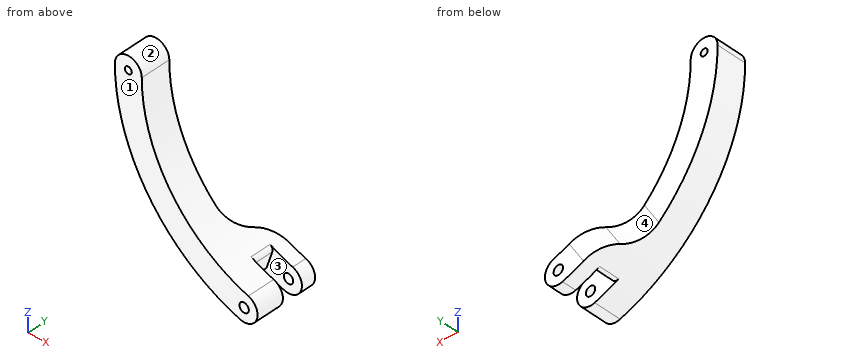
from build123d import *

# Parameters (mm, degrees)
SKETCH1_R               = 0.7499999999999986
SKETCH1_R_2             = 1.0249999999999995
BOSS_EXTRUDE1_DEPTH     = 6.510019999999999
BOSS_EXTRU_1_DEPTH      = 7.112
CONG_1_R                = 7.112
CONG_2_R                = 6.35
ENL_V_MAT_EXTRU_1_DEPTH = 4.444999999999999
ESQUISSE4_R             = 1.024999999999998
ENL_V_MAT_EXTRU_2_DEPTH = 57.18027536353634
CONG_3_R                = 1.016


with BuildPart() as part:
    # Sketch1 → Boss-Extrude1 (new body)
    with BuildSketch(Plane(origin=(0, 0, 0), x_dir=(1, 0, 0), z_dir=(0, 1, 0))):
        with BuildLine():
            ThreePointArc((-33.59051080682659, 0), (-27.195497439499345, 19.716169386615615), (-10.445442396451748, 31.92514916810793))
            ThreePointArc((-10.445442396451748, 31.92514916810793), (-8.576954256445317, 35.61090468912391), (-12.262709777461287, 37.4793928291303))
            ThreePointArc((-12.262709777461287, 37.4793928291303), (-31.926890187777666, 23.14633061338439), (-39.43448919317339, 0))
            ThreePointArc((-39.43448919317339, 0), (-36.512499999999996, -2.9219891931734026), (-33.59051080682659, 0))
        make_face()
        with Locations(Location((-36.512499999999996, 0, 0), (0, 0, 270))):
            Circle(SKETCH1_R, mode=Mode.SUBTRACT)
        with Locations(Location((-11.354076086956523, 34.702270998619134, 0), (0, 0, 270))):
            Circle(SKETCH1_R_2, mode=Mode.SUBTRACT)
    extrude(amount=BOSS_EXTRUDE1_DEPTH)

    # Esquisse1 → Boss.-Extru.1 (add)
    with BuildSketch(Plane(origin=(0, 6.510019999999999, 0), x_dir=(1, 0, 0), z_dir=(0, 1, 0))):
        with BuildLine():
            Line((-17.904180753250905, 28.421166897551096), (-21.0190975209346, 33.36579801731034))
            ThreePointArc((-21.0190975209346, 33.36579801731034), (-16.767530820930304, 35.69213986434075), (-12.262709777461293, 37.47939282913032))
            ThreePointArc((-12.262709777461293, 37.47939282913032), (-8.576954256445317, 35.610904689123906), (-10.44544239645175, 31.92514916810793))
            ThreePointArc((-10.44544239645175, 31.92514916810793), (-14.282673283409979, 30.40275744308238), (-17.904180753250905, 28.421166897551096))
        make_face()
    extrude(amount=BOSS_EXTRU_1_DEPTH)

    # Congé1
    cong_1_edges = [part.edges().sort_by_distance(p)[0] for p in [
        (-19.461639137092753, 6.510019999999999, -30.893482457430718),
    ]]
    fillet(cong_1_edges, radius=CONG_1_R - 0.0001)  # a hair under: the kernel refuses the full size

    # Congé2
    cong_2_edges = [part.edges().sort_by_distance(p)[0] for p in [
        (-19.461639137092753, 13.62202, -30.893482457430718),
    ]]
    fillet(cong_2_edges, radius=CONG_2_R)

    # Esquisse3 → Enlèv. mat.-Extru.1 (cut, symmetric)
    with BuildSketch(Plane(origin=(-12.262709777461295, 0, -37.479392829130326), x_dir=(0.3109640831758033, 0, 0.9504216637759433), z_dir=(-0.9504216637759433, 0, 0.3109640831758033))):
        Polygon((-5.92976249492949, 10.499999999999998), (8.153118343955157, 10.499999999999998), (8.153118343955159, 6), (-5.92976249492949, 6), align=None)
    extrude(amount=ENL_V_MAT_EXTRU_1_DEPTH, both=True, mode=Mode.SUBTRACT)

    # Esquisse4 → Enlèv. mat.-Extru.2 (cut, through all)
    with BuildSketch(Plane.XZ):
        with Locations(Location((-11.354076086956523, -34.702270998619134, 0), (0, 0, 270))):
            Circle(ESQUISSE4_R)
    extrude(amount=-ENL_V_MAT_EXTRU_2_DEPTH, mode=Mode.SUBTRACT)

    # Congé3
    cong_3_edges = [part.edges().sort_by_distance(p)[0] for p in [
        (-16.409183233920817, 8.25, -35.85829950683831),
        (-14.578207843975182, 8.25, -30.262159082282853),
    ]]
    fillet(cong_3_edges, radius=CONG_3_R)


solid = part.part
Work out the finished part from the listing and answer in its coordinate system (mm). Face numbers are marked on the shaded views. Give positions to 0.01 mm unless a question says otherwise; leave off trailing zeros. Loops run counter-clockwise (first coordinate to the right, second up) from the corner with the lowest first, then second, coordinate; pieces in that order, holes last. Notation, with made-up numbers: (59.5, 66.5) -> (89.5, 66.5) arc R28 cw to (89.5, 94.5) -> close; hole circle Ø7 at (-39.5, 74). An arc over 180 degrees is marked (long way). Use a Markdown table: item, result. Add a question column.
1. Determine the mould class of the marked faces 1, 2, 3 and 4 for opening direction Y: released by +Y, released by -Y, zero draft, split by the parting line, or undercut.
2. Find the intervals of material crossed by probe 1 along Y at (x, z) = (-35.5, -1.5); probe 2 along X at (y, z) = (12.25, -34); probe 3 along Z at (x, y) = (-10.5, 13), in increasing order.
3. Flat-ended cylindrical pins translate along their axes: pin 1 Ø5 at (y, z) = (4, -6.5) entering from +X; pin 2 Ø5 at (x, z) = (-35, -14.5) entering from +Y; pin 3 Ø2 at (x, y) = (-23.5, 8) entering from -Z; pin 4 Ø1.6 at (x, z) = (-11.35, -34.7) entering from +Y. Find the tip coordinate at first contact, or state that the pin passes through.
4. Section B-B on x = -38 is taken. Determine the outline of the cut face in (y, z).
5. Section A-A on y = 9.75 is taken. Determine the outline of the cut face in (x, z).
Results below:
| question | item | result |
|---|---|---|
| 1 | face 1 | released by -Y |
| 1 | face 2 | zero draft |
| 1 | face 3 | undercut |
| 1 | face 4 | released by +Y |
| 2 | probe 1 | y = 0 to 6.51 |
| 2 | probe 2 | x = -19.98 to -12.1, -10.61 to -8.52 |
| 2 | probe 3 | z = -37.5 to -35.27, -34.14 to -31.91 |
| 3 | pin 1 | stops at x = -32.36 |
| 3 | pin 2 | stops at y = 6.51 |
| 3 | pin 3 | stops at z = -32.39 |
| 3 | pin 4 | passes through |
| 4 | outline | (0, -10.54) -> (6.51, -10.54) -> (6.51, 2.52) -> (0, 2.52) -> close |
| 5 | outline | (-21.98, -32.74) arc R39.43 ccw to (-17.47, -35.36) arc R1.02 ccw to (-16.05, -34.76) -> (-14.85, -31.1) arc R1.02 ccw to (-15.35, -29.88) arc R33.59 cw to (-18.86, -27.79) -> close |
